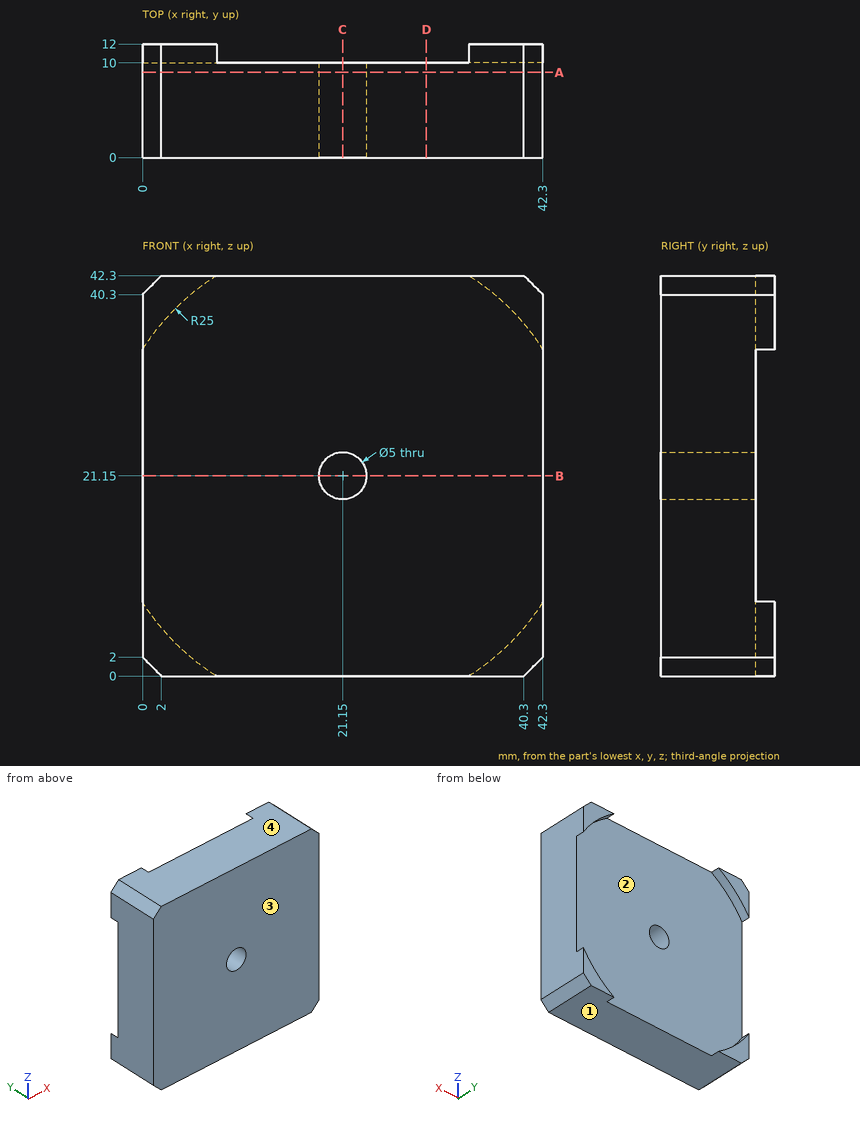
The figure shows three views and two pictorial views of one solid part (mm, origin at its lowest corner). Answer the questions. Give positions to 0.01 mm unless a question says otherwise; leave off trailing zeros. Loops run counter-clockwise (first coordinate to the right, second up) from the corner with the lowest first, then second, coordinate; pieces in that order, holes last. Notation, with made-up numbers: (73, 44) -> (103, 44) arc R20 ccw to (103, 81) -> close; hole circle Ø2 at (51, 28.25). An arc over 180 degrees is marked (long way). Use a Markdown table: item, result. Add a question column.
1. Find the intervals of material crossed by probe 1 along Z at (x, y) = (21.15, 5.5); probe 2 along Y at (x, z) = (34.5, 20.5), in increasing order.
2. Flat-ended cylindrical pins translate along their axes: pin 1 Ø12.5 at (x, z) = (16, 27) entering from +Y; pin 2 Ø6 at (x, z) = (19, 34) entering from -Y; pin 3 Ø4 at (x, z) = (21.15, 21.15) entering from -Y. Find the tip coordinate at first contact, or state that the pin passes through.
3. Determine the mould class of the marked faces 1, 2, 3 and 4 for opening direction Z: released by +Z, released by -Z, zero draft, split by the parting line, or undercut.
4. Section A-A on y = 9 is taken. Determine the outline of the cut face in (x, z).
5. Section B-B on z = 21.15 is taken. Determine the outline of the cut face in (x, y).
6. Section C-C on x = 21.15 is taken. Determine the outline of the cut face in (y, z), and give its area (3 significant figures).
7. Section D-D on x = 30 is taken. Determine the outline of the cut face in (y, z), and give its area (3 significant figures).
Results below:
| question | item | result |
|---|---|---|
| 1 | probe 1 | z = 0 to 18.65, 23.65 to 42.3 |
| 1 | probe 2 | y = 0 to 10 |
| 2 | pin 1 | stops at y = 10 |
| 2 | pin 2 | stops at y = 0 |
| 2 | pin 3 | passes through |
| 3 | face 1 | released by -Z |
| 3 | face 2 | undercut |
| 3 | face 3 | zero draft |
| 3 | face 4 | released by +Z |
| 4 | outline | (0, 2) -> (2, 0) -> (40.3, 0) -> (42.3, 2) -> (42.3, 40.3) -> (40.3, 42.3) -> (2, 42.3) -> (0, 40.3) -> close; hole circle Ø5 at (21.15, 21.15) |
| 5 | outline | (0, 0) -> (18.65, 0) -> (18.65, 10) -> (0, 10) -> close; (23.65, 0) -> (42.3, 0) -> (42.3, 10) -> (23.65, 10) -> close |
| 6 | outline | (0, 0) -> (10, 0) -> (10, 18.65) -> (0, 18.65) -> close; (0, 23.65) -> (10, 23.65) -> (10, 42.3) -> (0, 42.3) -> close |
| 6 | area | 373 mm^2 |
| 7 | outline | (0, 0) -> (10, 0) -> (10, 42.3) -> (0, 42.3) -> close |
| 7 | area | 423 mm^2 |
